Geometry: final body of the model. Coordinates: model frame, mm. A direction names the side the tool comes from. Coordinates: 2 decimals unless noted, no trailing zeros. Loops run counter-clockwise (first coordinate to the right, second up) from the corner with the lowest first, then second, coordinate; pieces in that order, holes last. Notation, with made-up numbers: (-35.5, -14.75) -> (20.5, -14.75) arc R32 ccw to (20.5, 20.25) -> close; hole circle Ø7 at (-28.5, 79.25). An arc over 180 degrees is marked (long way). One line per item, written item: value. Start each with the question number.
Autodesk Inventor part; units mm, degrees
ref_plane "Start plane" through (0, 0, -20) normal (0, 0, 1) x (1, 0, 0)
ref_plane "End plane" through (0, 0, 720) normal (0, 0, 1) x (1, 0, 0)
ref_plane "Work Plane4" through (0, -20, -20) normal (0, 0.7071, -0.7071) x (1, 0, 0)
ref_plane "Start plane" through (0, 0, -20) normal (0, 0, 1) x (1, 0, 0)
ref_plane "End plane" through (0, 0, 720) normal (0, 0, 1) x (1, 0, 0)
sketch "Sketch" plane through (0, 0, 0) normal (0, 0, 1) x (1, 0, 0)
  line L0 (-20, -16) -> (-20, 16)
  line L1 (-16, 20) -> (16, 20)
  line L2 (20, 16) -> (20, -16)
  line L3 (16, -20) -> (-16, -20)
  arc A0 (-20, -16) -> (-16, -20) centre (-16, -16) ccw
  arc A1 (20, 16) -> (16, 20) centre (16, 16) ccw
  arc A2 (-16, 20) -> (-20, 16) centre (-16, 16) ccw
  arc A3 (16, -20) -> (20, -16) centre (16, -16) ccw
  arc A4 (-16, 18) -> (-18, 16) centre (-16, 16) ccw
  line L4 (-16, 18) -> (16, 18)
  arc A5 (18, 16) -> (16, 18) centre (16, 16) ccw
  line L5 (18, 16) -> (18, -16)
  arc A6 (16, -18) -> (18, -16) centre (16, -16) ccw
  line L6 (16, -18) -> (-16, -18)
  arc A7 (-18, -16) -> (-16, -18) centre (-16, -16) ccw
  line L7 (-18, -16) -> (-18, 16)
  line L8 (0, 29.1598) -> (0, -29.1598) construction
  line L9 (-29.1598, 0) -> (29.1598, 0) construction
  dimension "d7" = 4
  dimension "d9" = 40
  dimension "d11" = 40
  dimension "d12" = 2
  dimension "d15" = 20
  dimension "d16" = 20
extrude "Body" add sketch "Sketch" along normal up to surface (740 mm away) from surface at -20
sketch "Sketch3" plane through (0, 0, 0) normal (0, 0, 1) x (1, 0, 0)
  line L0 (0, 0) -> (10, 0)
ref_plane "Work Plane3" through (0, 0, 0) normal (0, -1, 0) x (1, 0, 0)
sketch "Sketch4" plane through (0, 0, 0) normal (0, -1, 0) x (1, 0, 0)
  line L0 (-2, -20) -> (12, -20)
  line L1 (-2, 720) -> (12, 720)
  dimension "d18" = 740
ref_plane "Work Plane4" through (0, -20, -20) normal (0, 0.7071, -0.7071) x (1, 0, 0)
split "Split1" plane through (0, -20, -20) removes the side toward (0, 0.7071, -0.7071)
ref_plane "Work Plane5" through (0, -20, 720) normal (0, 0.7071, 0.7071) x (1, 0, 0)
split "Split2" plane through (0, -20, 720) removes the side toward (0, 0.7071, 0.7071)
equation "\"d7\" = G_IR"
equation "\"d9\" = G_W"
equation "\"d11\" = G_H"
equation "\"d12\" = G_T"
equation "\"d15\" = 0.5 * d9"
equation "\"d16\" = 0.5 * d11"
equation "\"d3\" = G_L"
equation "\"G_W\" = 40"
equation "\"G_H\" = 40"
equation "\"G_T\" = 2"
equation "\"G_IR\" = 4"
equation "\"G_L\" = d18"
equation "\"G_OFFSET_START\" = 20"
equation "\"G_OFFSET_END\" = 20"
equation "\"d13\" = -G_OFFSET_START"
equation "\"d14\" = G_OFFSET_END + B_L"
equation "\"B_L\" = 700"
properties part number "ISO 4019 - 40x40x2 - 740" material "Steel, Mild"
1. Draft query along X for faces 1 (the face through (-18, 0, 345)), 2 (the face through (18, 0, 345)), 3 (the face through (-20, 0, 345)), 4 (the face through (20, 0, 345)). Return one class per face: released by +X, released by -X, zero draft, split by the parting line, or undercut.
2. Pin query (flat end, axial travel): pin 1 Ø8 at (x, y) = (15, 4.5) entering from -Z. Return the tip coordinate at first contact, or that it passes through.
3. Line query: L1, parallel to Y at x = 11.5, z = 179; L2, parallel to X at y = 16.5, z = 383. Output: solid intervals per line, ascending. Write a range as [from, to].
4. Section C-C on y = -0.5. Return the cut outline in (x, z), plus the area to 3 significant figures.
5. Section B-B on z = 610.5. Return the cut outline in (x, y).
6. Section A-A on x = -6.5. Return the cut outline in (y, z).
7. Set-up query: faces 5 (the face through (19, -2, 702)), 6 (the face through (0, 18, 345)). Return all of +Z, -Z, +X, -X, +Y, -Y with unobstructed straight access to the full face (end or side cutting, diameter ignored); none if empty.
Checks:
1. face 1: undercut
1. face 2: undercut
1. face 3: released by -X
1. face 4: released by +X
2. pin 1: z = 1.85
3. L1: [-20, -18], [18, 20]
3. L2: [-19.97, -17.94], [17.94, 19.97]
4. outline: (-20, -0.5) -> (-18, -0.5) -> (-18, 700.5) -> (-20, 700.5) -> close; (18, -0.5) -> (20, -0.5) -> (20, 700.5) -> (18, 700.5) -> close
4. area: 2,800 mm²
5. outline: (-20, -16) arc R4 ccw to (-16, -20) -> (16, -20) arc R4 ccw to (20, -16) -> (20, 16) arc R4 ccw to (16, 20) -> (-16, 20) arc R4 ccw to (-20, 16) -> close; hole (-18, -16) arc R2 ccw to (-16, -18) -> (16, -18) arc R2 ccw to (18, -16) -> (18, 16) arc R2 ccw to (16, 18) -> (-16, 18) arc R2 ccw to (-18, 16) -> close
6. outline: (-20, -20) -> (-18, -18) -> (-18, 718) -> (-20, 720) -> close; (18, 18) -> (20, 20) -> (20, 680) -> (18, 682) -> close
7. face 5: +Z, +X, -X, +Y
7. face 6: +Z, -Z
